```python
from build123d import *

# Parameters (mm, degrees)
RESSALTO_EXTRUS_O1_DEPTH = 75
RESSALTO_EXTRUS_O2_DEPTH = 40
ESBO_O4_W                = 10
ESBO_O4_H                = 30
RESSALTO_EXTRUS_O3_DEPTH = 35
CORTE_EXTRUS_O1_REACH    = 101.247


with BuildPart() as part:
    # Esboço2 → Ressalto-extrusão1 (new body)
    with BuildSketch(Plane.XY):
        Polygon((-60, 35), (-60, 0), (0, 0), (0, 65), (-25, 65), (-25, 35), align=None)
    extrude(amount=-RESSALTO_EXTRUS_O1_DEPTH)

    # Esboço3 → Ressalto-extrusão2 (add)
    with BuildSketch(Plane(origin=(0, 0, 0), x_dir=(0, 0, -1), z_dir=(1, 0, 0))):
        with BuildLine():
            Line((65, 65), (51.71553286, 43.412740898))
            ThreePointArc((51.71553286, 43.412740898), (32.225125249, 37.861461385), (36.052707483, 17.96064966))
            Line((36.052707483, 17.96064966), (25, 0))
            Line((25, 0), (75, 0))
            Line((75, 0), (75, 65))
            Line((75, 65), (65, 65))
        make_face()
    extrude(amount=RESSALTO_EXTRUS_O2_DEPTH)

    # Esboço4 → Ressalto-extrusão3 (add)
    with BuildSketch(Plane.ZY.offset(25)):
        with Locations((-35, 50)):
            Rectangle(ESBO_O4_W, ESBO_O4_H)
    extrude(amount=RESSALTO_EXTRUS_O3_DEPTH)

    # Esboço6 → Corte-extrusão1 (cut, up to next)
    with BuildSketch(Plane.XY.offset(-30), mode=Mode.PRIVATE) as corte_extrus_o1_sk1:
        Polygon((-25, 65), (-60, 35), (-60, 65), align=None)
    corte_extrus_o1_tool1 = extrude(corte_extrus_o1_sk1.sketch, amount=-CORTE_EXTRUS_O1_REACH, mode=Mode.PRIVATE) & part.part
    add(corte_extrus_o1_tool1.solids().sort_by_distance((-48.333333, 55, -30))[0], mode=Mode.SUBTRACT)


solid = part.part
```
Can you work these out from the model? Positions are in its coordinate system, mm. A direction names the side the tool comes from. Coordinates: 2 decimals unless noted, no trailing zeros. Order: outer loops, then holes, each group sorted by start corner. A loop starts at its lowest first (then second) coordinate and runs counter-clockwise, first axis right, second up. Notation, with made-up numbers: (-26.5, 35.25) - (23.5, 35.25) arc R23 cw to (23.5, 69.25) - close; hole circle Ø10 at (-23.75, 70). An arc over 180 degrees is marked (long way). Answer in a Markdown table with one row per item.
1. If I drill on line 1 along X through (y, z) = (38, -72); line 2 along Z through (x, y) = (14.5, 43.5); line 3 along Y through (x, z) = (-53, -44), over which ranges is the centre line in solid material (lowest first)?
Reply:
| item | result |
|---|---|
| line 1 | x = -25 to 40 |
| line 2 | z = -75 to -51.77, -51.54 to -38.46 |
| line 3 | y = 0 to 35 |
2. Suppose I cut it at B-B (x = 17). Please give me the cut outline in (y, z).
Reply:
| item | result |
|---|---|
| outline | (0, -75) - (65, -75) - (65, -65) - (43.41, -51.72) arc R15 ccw to (17.96, -36.05) - (0, -25) - close |
3. Suppose I cut it at D-D (y = 59.5). Please give me the cut outline in (x, z).
Reply:
| item | result |
|---|---|
| outline | (-31.42, -40) - (-25, -40) - (-25, -75) - (40, -75) - (40, -61.62) - (0, -61.62) - (0, 0) - (-25, 0) - (-25, -30) - (-31.42, -30) - close |
4. Suppose I cut it at C-C (y = 21). Please give me the cut outline in (x, z), and give its area (3 significant figures).
Reply:
| item | result |
|---|---|
| outline | (-60, -75) - (40, -75) - (40, -33) - (0, -33) - (0, 0) - (-60, 0) - close |
| area | 6,180 mm^2 |
5. For pin 1 (15 mm diameter, centred on x = -39.5, y = 52, fed in from +Z); pin 2 (15 mm diameter, centred on y = 48, z = -18.5, fed in from -X); pin 3 (1 mm diameter, centred on x = -34.5, z = -61, fed in from +Y), each with a flat end and sliding along its axis, tell me the tip position at first contact or that it passes through.
Reply:
| item | result |
|---|---|
| pin 1 | stops at z = -30 |
| pin 2 | stops at x = -25 |
| pin 3 | stops at y = 35 |
6. Suppose I cut it at A-A (z = -27.5). Please give me the cut outline in (x, y).
Reply:
| item | result |
|---|---|
| outline | (-60, 0) - (40, 0) - (40, 4.06) - (0, 4.06) - (0, 65) - (-25, 65) - (-25, 35) - (-60, 35) - close |
7. For faces 1 (the flat face through (-25, 50, -57)), 2 (the flat face through (-25, 50, -15)), 3 (the flat face through (19.7, 9.1, -30.6)), which set-ups out of +Z, -Z, +X, -X, +Y, -Y let a thin tool reach every point of the face, with its end or its side?
Reply:
| item | result |
|---|---|
| face 1 | -Z, -X, +Y |
| face 2 | +Z, -X, +Y |
| face 3 | +Z, +X |
